Can you work these out from the model? Positions are in its coordinate system, mm. Face numbers are marked on the shaded views. A direction names the side the tool comes from. Give positions to 0.01 mm unless a question says otherwise; leave off trailing zeros. Order: outer loops, then holes, each group sorted by start corner. A loop starts at its lowest first (then second) coordinate and runs counter-clockwise, first axis right, second up. Notation, with made-up numbers: (-39, 49.25) - (-28, 49.25) arc R28 ccw to (-28, 75.25) - close; hole circle Ø11 at (53, 39.25). An arc over 180 degrees is marked (long way). Use one line per item in the form item = value. Start each with the question number.
1) For pin 1 (8 mm diameter, centred on x = 85, y = 32.5, fed in from -Z); pin 2 (3.5 mm diameter, centred on y = 137.5, z = -1.5, fed in from +X); pin 3 (1.5 mm diameter, centred on x = 25, z = -21, fed in from +Y); pin 4 (3.5 mm diameter, centred on x = 123, z = -24.5, fed in from -Y), each with a flat end and sliding along its axis, tell me the tip position at first contact or that it passes through.
2) Suppose I cut it at C-C, the plane x = -70. Write out the boundary of the cut face in (y, z).
3) Suppose I cut it at D-D, the plane y = 40. Write out the boundary of the cut face in (x, z).
4) We'd pull the mould along X, two halves only. Please class the marked faces 3, 4 and 5: released by +X, released by -X, zero draft, split by the parting line, or undercut.
5) Which directions (+Z, -Z, +X, -X, +Y, -Y) give clear straight access to the entire face, cutting with the end or side of a thin tool? Please do the marked faces 1 and 2.
6) Suppose I cut it at A-A, the plane x = 0. Write out the boundary of the cut face in (y, z).
7) Please list where these lines run through material, in increasing order: probe 1 along Y at (x, z) = (70, -1); probe 2 along X at (y, z) = (147, -10.5); probe 3 along X at (y, z) = (180, -2.1).
8) Suppose I cut it at B-B, the plane y = 96.5. Write out the boundary of the cut face in (x, z), and give its area (3 significant figures).
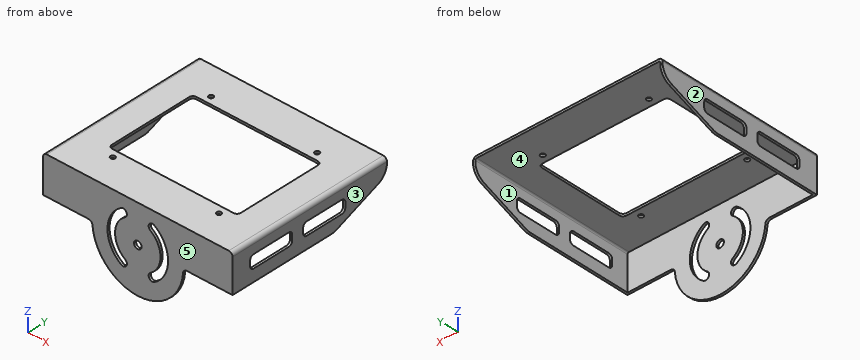
```python
from build123d import *

# Parameters (mm, degrees)
F7_DEPTH  = 220
F8_DEPTH  = 3
F9_DEPTH  = 3
F0_R      = 5
F10_DEPTH = 3
F11_R     = 5
F12_R     = 5
F13_R     = 3
F14_DEPTH = 25


with BuildPart() as f7:
    # F4 (on offset) → F7 (new body)
    with BuildSketch(Plane.XZ.offset(-220)):
        with BuildLine():
            Line((125, -6.430699), (125, -2))
            ThreePointArc((125, -2), (124.414214, -0.585786), (123, 0))
            Line((123, 0), (-123, 0))
            ThreePointArc((-123, 0), (-124.414214, -0.585786), (-125, -2))
            Line((-125, -2), (-125, -6.430699))
            Line((-125, -6.430699), (-122, -6.430699))
            Line((-122, -6.430699), (-122, -5))
            ThreePointArc((-122, -5), (-121.414214, -3.585786), (-120, -3))
            Line((-120, -3), (120, -3))
            ThreePointArc((120, -3), (121.414214, -3.585786), (122, -5))
            Line((122, -5), (122, -6.430699))
            Line((122, -6.430699), (125, -6.430699))
        make_face()
    extrude(amount=F7_DEPTH)

    # F6 (on offset) → F8 (join)
    with BuildSketch(Plane.YZ.offset(-125)):
        with BuildLine():
            Line((220, -6.430699), (220, 0))
            Line((220, 0), (0, 0))
            Line((0, 0), (0, -50))
            Line((0, -50), (140.739724, -50))
            ThreePointArc((140.739724, -50), (144.5026, -49.64283), (148.131078, -48.584076))
            Line((148.131078, -48.584076), (207.391354, -25.014775))
            ThreePointArc((207.391354, -25.014775), (216.550334, -17.659522), (220, -6.430699))
        make_face()
        with BuildLine():
            ThreePointArc((25, -22), (26.464466, -18.464466), (30, -17))
            Line((30, -17), (80, -17))
            ThreePointArc((80, -17), (83.535534, -18.464466), (85, -22))
            Line((85, -22), (85, -29))
            ThreePointArc((85, -29), (83.535534, -32.535534), (80, -34))
            Line((80, -34), (30, -34))
            ThreePointArc((30, -34), (26.464466, -32.535534), (25, -29))
            Line((25, -29), (25, -22))
        make_face(mode=Mode.SUBTRACT)
        with BuildLine():
            ThreePointArc((100.627564, -22), (102.09203, -18.464466), (105.627564, -17))
            Line((105.627564, -17), (155.627564, -17))
            ThreePointArc((155.627564, -17), (159.163098, -18.464466), (160.627564, -22))
            Line((160.627564, -22), (160.627564, -29))
            ThreePointArc((160.627564, -29), (159.163098, -32.535534), (155.627564, -34))
            Line((155.627564, -34), (105.627564, -34))
            ThreePointArc((105.627564, -34), (102.09203, -32.535534), (100.627564, -29))
            Line((100.627564, -29), (100.627564, -22))
        make_face(mode=Mode.SUBTRACT)
    extrude(amount=F8_DEPTH)

    # F2 (on offset) → F9 (join)
    with BuildSketch(Plane.YZ.offset(125)):
        with BuildLine():
            Line((220, 0), (0, 0))
            Line((0, 0), (0, -50))
            Line((0, -50), (140.739724, -50))
            ThreePointArc((140.739724, -50), (144.5026, -49.64283), (148.131078, -48.584076))
            Line((148.131078, -48.584076), (207.391354, -25.014775))
            ThreePointArc((207.391354, -25.014775), (216.550334, -17.659522), (220, -6.430699))
            Line((220, -6.430699), (220, 0))
        make_face()
        with BuildLine():
            ThreePointArc((25, -22), (26.464466, -18.464466), (30, -17))
            Line((30, -17), (80, -17))
            ThreePointArc((80, -17), (83.535534, -18.464466), (85, -22))
            Line((85, -22), (85, -29))
            ThreePointArc((85, -29), (83.535534, -32.535534), (80, -34))
            Line((80, -34), (30, -34))
            ThreePointArc((30, -34), (26.464466, -32.535534), (25, -29))
            Line((25, -29), (25, -22))
        make_face(mode=Mode.SUBTRACT)
        with BuildLine():
            ThreePointArc((100.627564, -22), (102.09203, -18.464466), (105.627564, -17))
            Line((105.627564, -17), (155.627564, -17))
            ThreePointArc((155.627564, -17), (159.163098, -18.464466), (160.627564, -22))
            Line((160.627564, -22), (160.627564, -29))
            ThreePointArc((160.627564, -29), (159.163098, -32.535534), (155.627564, -34))
            Line((155.627564, -34), (105.627564, -34))
            ThreePointArc((105.627564, -34), (102.09203, -32.535534), (100.627564, -29))
            Line((100.627564, -29), (100.627564, -22))
        make_face(mode=Mode.SUBTRACT)
    extrude(amount=-F9_DEPTH)

    # F0 (on Front) → F10 (join)
    with BuildSketch(Plane.XZ):
        with BuildLine():
            ThreePointArc((-64.807407, -50), (-61.410576, -51.331003), (-59.822222, -54.615385))
            ThreePointArc((-59.822222, -54.615385), (0, -110), (59.822222, -54.615385))
            ThreePointArc((59.822222, -54.615385), (61.410576, -51.331003), (64.807407, -50))
            Line((64.807407, -50), (125, -50))
            Line((125, -50), (125, 0))
            Line((125, 0), (-125, 0))
            Line((-125, 0), (-125, -50))
            Line((-125, -50), (-64.807407, -50))
        make_face()
        with BuildLine():
            ThreePointArc((-16.583124, -25), (-30, -50), (-16.583124, -75))
            ThreePointArc((-16.583124, -75), (-15.180311, -81.930521), (-22.110832, -83.333333))
            ThreePointArc((-22.110832, -83.333333), (-40, -50), (-22.110832, -16.666667))
            ThreePointArc((-22.110832, -16.666667), (-15.180311, -18.069479), (-16.583124, -25))
        make_face(mode=Mode.SUBTRACT)
        with Locations((0, -50)):
            Circle(F0_R, mode=Mode.SUBTRACT)
        with BuildLine():
            ThreePointArc((22.110832, -83.333333), (15.180311, -81.930521), (16.583124, -75))
            ThreePointArc((16.583124, -75), (30, -50), (16.583124, -25))
            ThreePointArc((16.583124, -25), (15.180311, -18.069479), (22.110832, -16.666667))
            ThreePointArc((22.110832, -16.666667), (40, -50), (22.110832, -83.333333))
        make_face(mode=Mode.SUBTRACT)
    extrude(amount=-F10_DEPTH)

    # F11
    f11_edges = [f7.edges().sort_by_distance(p)[0] for p in [
        (125, 110, 0),
    ]]
    fillet(f11_edges, radius=F11_R)

    # F12
    f12_edges = [f7.edges().sort_by_distance(p)[0] for p in [
        (-125, 110, 0),
    ]]
    fillet(f12_edges, radius=F12_R)

    # F13 (on face) → F14 (cut)
    with BuildSketch(Plane.XY):
        with BuildLine():
            Line((-80, 50), (80, 50))
            ThreePointArc((80, 50), (83.535534, 51.464466), (85, 55))
            Line((85, 55), (85, 165))
            ThreePointArc((85, 165), (83.535534, 168.535534), (80, 170))
            Line((80, 170), (-80, 170))
            ThreePointArc((-80, 170), (-83.535534, 168.535534), (-85, 165))
            Line((-85, 165), (-85, 55))
            ThreePointArc((-85, 55), (-83.535534, 51.464466), (-80, 50))
        make_face()
        with Locations((-70, 180)):
            Circle(F13_R)
        with Locations((-70, 40)):
            Circle(F13_R)
        with Locations((70, 40)):
            Circle(F13_R)
        with Locations((70, 180)):
            Circle(F13_R)
    extrude(amount=-F14_DEPTH, mode=Mode.SUBTRACT)


solid = f7.part
```
Result sheet:
q1.pin_1 = -3
q1.pin_2 = 124.68
q1.pin_3 = through
q1.pin_4 = 0
q2.outline = (0, -50) - (3, -50) - (3, -3) - (37, -3) - (37, 0) - (0, 0) - close; (43, -3) - (50, -3) - (50, 0) - (43, 0) - close; (170, -3) - (177, -3) - (177, 0) - (170, 0) - close; (183, -3) - (220, -3) - (220, 0) - (183, 0) - close
q3.outline = (-125, -50) - (-122, -50) - (-122, -34) - (-125, -34) - close; (-125, -17) - (-122, -17) - (-122, -5) arc R2 cw to (-120, -3) - (-73, -3) - (-73, 0) - (-120, 0) arc R5 ccw to (-125, -5) - close; (-67, -3) - (67, -3) - (67, 0) - (-67, 0) - close; (73, -3) - (120, -3) arc R2 cw to (122, -5) - (122, -17) - (125, -17) - (125, -5) arc R5 ccw to (120, 0) - (73, 0) - close; (122, -50) - (125, -50) - (125, -34) - (122, -34) - close
q4.face_3 = released by +X
q4.face_4 = undercut
q4.face_5 = zero draft
q5.face_1 = -Z, +Y
q5.face_2 = +Z, -Z, -X, +Y, -Y
q6.outline = (0, -110) - (3, -110) - (3, -55) - (0, -55) - close; (0, -45) - (3, -45) - (3, -3) - (50, -3) - (50, 0) - (0, 0) - close; (170, -3) - (220, -3) - (220, 0) - (170, 0) - close
q7.probe_1 = 0 to 37, 43 to 50, 170 to 177, 183 to 220
q7.probe_2 = -125 to -122, 122 to 125
q7.probe_3 = -124.07 to -73, -67 to 67, 73 to 124.07
q8.outline = (-125, -50) - (-122, -50) - (-122, -5) arc R2 cw to (-120, -3) - (-85, -3) - (-85, 0) - (-120, 0) arc R5 ccw to (-125, -5) - close; (85, -3) - (120, -3) arc R2 cw to (122, -5) - (122, -50) - (125, -50) - (125, -5) arc R5 ccw to (120, 0) - (85, 0) - close
q8.area = 513 mm²
